Study the drawing (mm; zero at the part's minimum x, y, z) and answer. A direction names the side the tool comes from. Give positions to 0.01 mm unless a question says otherwise; leave off trailing zeros. Write each loop counter-clockwise with the first axis right and the second up, starting at its lowest first coordinate (ties: lowest second). Pieces come first, ordered by that corner, then holes. Notation, with made-up numbers: (-6, 5.25) - (7, 5.25) arc R25 cw to (7, 36.25) - close; hole circle Ø4 at (5.5, 59). An arc over 180 degrees is marked (long way). Return JSON: item names as keys, results as strings.
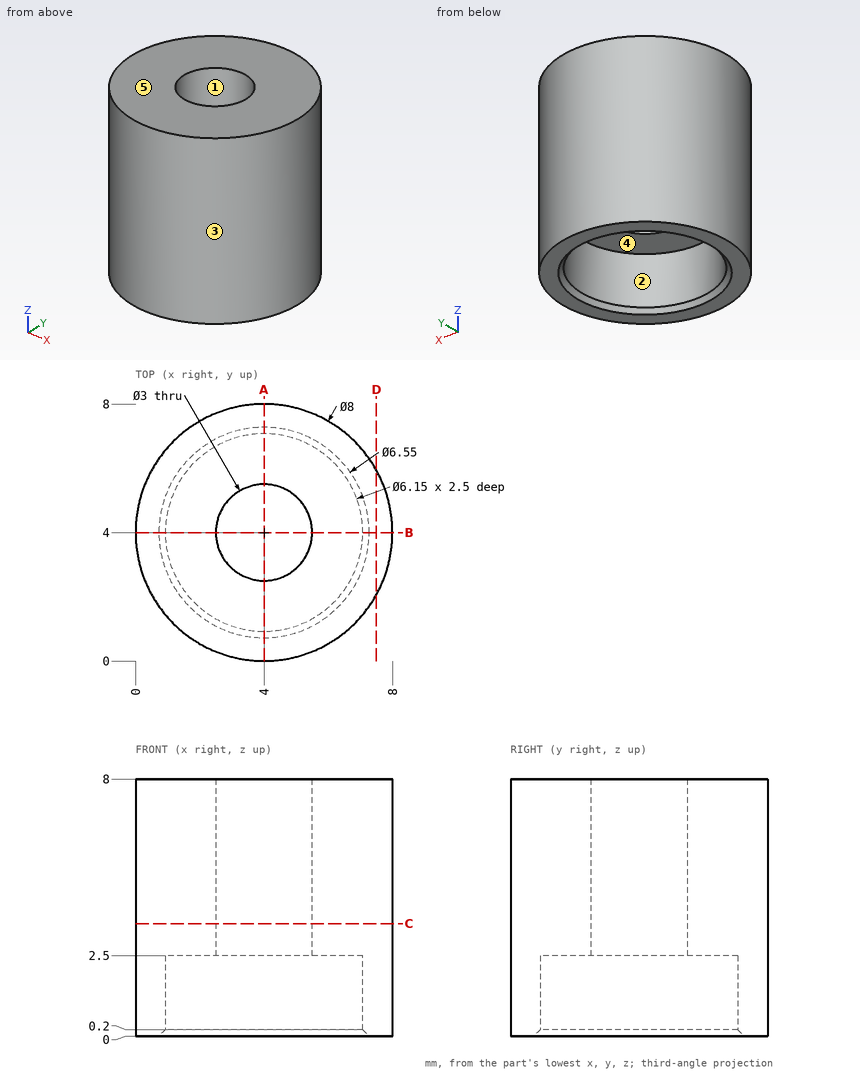
Item 1: A cutting plane is placed at A-A on x = 4. Determine the outline of the cut face in (y, z) (3 decimals), then the cut area to 3 significant figures.
Answer below:
{"outline": "(0, 0) - (0.725, 0) - (0.925, 0.2) - (0.925, 2.5) - (2.5, 2.5) - (2.5, 8) - (0, 8) - close; (5.5, 2.5) - (7.075, 2.5) - (7.075, 0.2) - (7.275, 0) - (8, 0) - (8, 8) - (5.5, 8) - close", "area": "32.1 mm²"}
Item 2: The mould has two halves that part along Y. Classify the marked faces 3, 4 and 5: +Y half, -Y half, draft (parallel to the pull), parting line (faces both ways), or undercut.
Answer below:
{"face 3": "parting line", "face 4": "undercut", "face 5": "draft"}
Item 3: A cutting plane is placed at D-D on x = 7.5. Determine the outline of the cut face in (y, z).
Answer below:
{"outline": "(2.06, 0) - (5.94, 0) - (5.94, 8) - (2.06, 8) - close"}
Item 4: A cutting plane is placed at C-C on z = 3.5. Determine the outline of the cut face in (x, y), then the cut area to 3 significant figures.
Answer below:
{"outline": "circle Ø8 at (4, 4); hole circle Ø3 at (4, 4)", "area": "43.2 mm²"}
Item 5: Flat-ended cylindrical pins translate along their axes: P1, Ø4, axis at x = 7, z = 5.5, coming from the -Y side; P2, Ø3.5, axis at x = 4, y = 4, coming from the -Z side; P3, Ø1, axis at x = 6.5, z = 6, coming from the -Y side. Find the tip coordinate at first contact, or state that the pin passes through.
Answer below:
{"P1": "stops at y = 0.13", "P2": "stops at z = 2.5", "P3": "stops at y = 0.54"}
Item 6: For the marked faces 1 and 2, determine the directions among +Z, -Z, +X, -X, +Y, -Y from which every point of the face is accessible in a straight line to the end or side of a thin tool.
Answer below:
{"face 1": "+Z, -Z", "face 2": "-Z"}
Item 7: Consider L1, parallel to Y at x = 4, z = 1.7 (3 decimals); L2, parallel to Y at x = 4, z = 5.1; L3, parallel to Z at x = 3.75, y = 1.5. Determine where each line is inside the solid, lowest interval first.
Answer below:
{"L1": "y = 0 to 0.925, 7.075 to 8", "L2": "y = 0 to 2.5, 5.5 to 8", "L3": "z = 2.5 to 8"}
